Study the drawing (mm; zero at the part's minimum x, y, z) and answer. A direction names the side the tool comes from. Coordinates: 2 decimals unless noted, no trailing zeros. Loops run counter-clockwise (first coordinate to the right, second up) from the corner with the lowest first, then second, coordinate; pieces in that order, holes last. Notation, with made-up numbers: (-34.75, -32.75) -> (2.25, -32.75) arc R35 ccw to (2.25, 2.25) -> close; hole circle Ø11 at (26.25, 66). An arc over 180 degrees is marked (long way). Answer as a JSON object with one key per item and string values. Group by question number.
Q1. Each of these flat-tipped pins is pushed along its axis until it touches: P1, Ø1, axis at y = 4.5, z = 49.5, coming from the -X side; P2, Ø1.5, axis at x = 76, z = 30, coming from the +Y side (1 decimal). Where does it stop, or does it pass through?
Q2. The part is cut by section A-A on z = 41. State how many separate pieces and enclosed holes the cut face has.
Q3. Determine the mould class of the marked faces 3, 4 and 5 for opening direction X: released by +X, released by -X, zero draft, split by the parting line, or undercut.
Q4. The part is cut by section D-D on z = 27.5. Write down the section's boundary in (x, y) (1 decimal).
Q5. Straight lines are drawn through the part: line 1 along Z through (x, y) = (38.5, 5); line 2 along X through (y, z) = (5, 36.5) (1 decimal); line 3 along Y through (x, z) = (92, 41) (1 decimal). For each, find the intervals that lie inside material, in ascending order. Write a range as [from, to].
Q6. For the marked faces 1 and 2, determine the directions among +Z, -Z, +X, -X, +Y, -Y from which every point of the face is accessible in a straight line to the end or side of a thin tool.
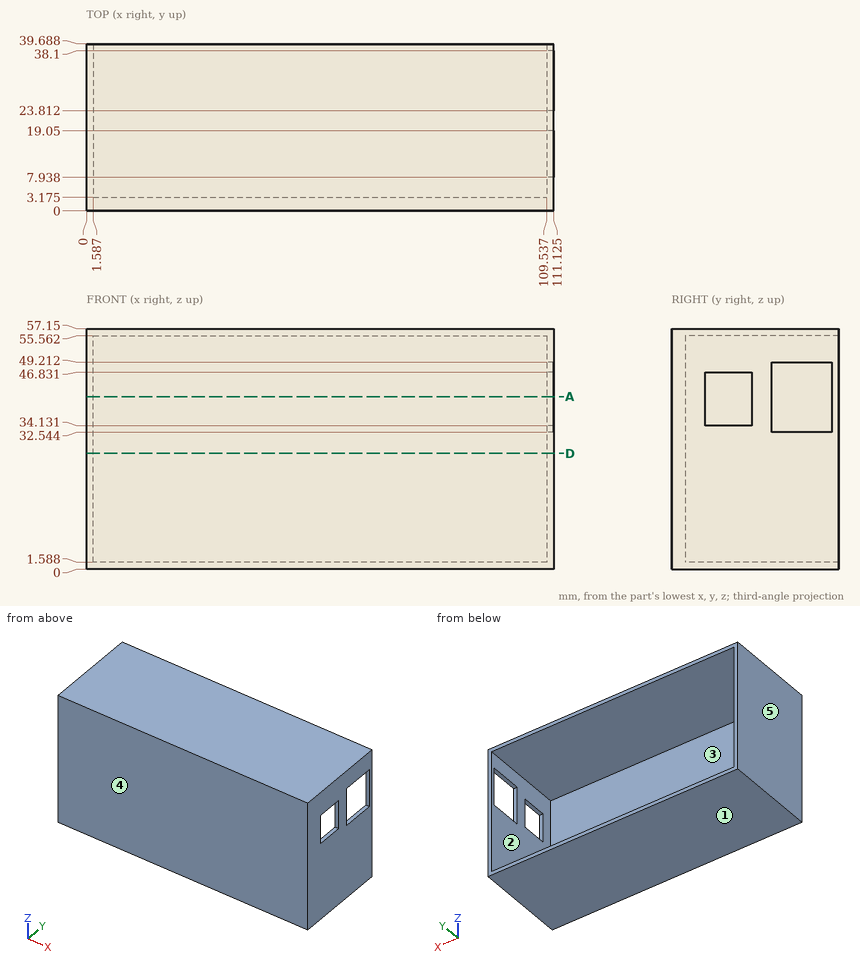
Final values:
{
 "1": {"P1": "stops at x = 0", "P2": "stops at y = 3.2"},
 "2": {"separate pieces": "3", "enclosed holes": "0"},
 "3": {"face 3": "undercut", "face 4": "zero draft", "face 5": "released by -X"},
 "4": {"outline": "(0, 0) -> (111.1, 0) -> (111.1, 39.7) -> (109.5, 39.7) -> (109.5, 3.2) -> (1.6, 3.2) -> (1.6, 39.7) -> (0, 39.7) -> close"},
 "5": {"line 1": "z = [0, 1.59], [55.56, 57.15]", "line 2": "x = [0, 1.6], [109.5, 111.1]", "line 3": "y = [0, 3.2]"},
 "6": {"face 1": "-Z, +X, -X, +Y, -Y", "face 2": "+Y"}
}
